Model file for the job. Use its own axes, mm. A direction names the side the tool comes from. Round coordinates to 2 decimals unless told otherwise and drop trailing zeros. Loops run counter-clockwise (first coordinate to the right, second up) from the corner with the lowest first, then second, coordinate; pieces in that order, holes last. Notation, with made-up numbers: M 88.5,49.5 L 142.5,49.5 A16 cw 142.5,69.5 Z; hole C 15,17.25 d2. An arc over 180 degrees is marked long. Use a Markdown table: item, result. Add a question column.
Q1. Tool access for faces 1 (the face through (0.3, 43.5, 32.414)), 2 (the face through (45, 0, 50)): list every direction of +Z, -Z, +X, -X, +Y, -Y with a clear straight run to the whole face (end or side of a thin tool).
Q2. Cut at B-B (y = -0.5). Give the cut face in (x, z), plus the area to 3 significant figures.
Q3. Pin check, flat tips, straight feed: pin 1 (8 mm diameter, centred on x = 15, y = 15, fed in from +Z); pin 2 (8 mm diameter, centred on x = 37.5, z = 42, fed in from -Y); pin 3 (13.5 mm diameter, centred on y = 40.5, z = 21, fed in from +X). Stop position of each tip, or through.
Q4. Cut at C-C (y = 62). Give the cut face in (x, z), plus the area to 3 significant figures.
Q5. Cut at D-D (z = 4.5). Give the cut face in (x, y), plus the area to 3 significant figures.
Q6. Cut at A-A (x = 0). Give the cut face in (y, z).
Q7. Mould opens along Y. For faces 3 (the face through (16.7, 75.7, 24)), 4 (the face through (-2.71, 44.434, 23.959)), 5 (the face through (-21.187, 46, 24)) say: +Y half, -Y half, draft (parallel to the pull), parting line (faces both ways), or undercut.
Q8. Probe line 1 (Y direction, x = 0, z = 27); line 2 (Y direction, x = 0, z = 19); line 3 (Y direction, x = -2, z = 35.5) (3 decimals). List the from-to ranges inside material, lowest first. Write a range as from..to.
from build123d import *

# Parameters (mm, degrees)
F0_W         = 100
F0_H         = 60
F1_DEPTH     = 60
F2_W         = 42.3733331263
F2_H         = 17.1486828476
F3_DEPTH     = 50
F4_R         = 12.5
F5_DEPTH     = 32.4145003611
F6_T1_DEPTH  = 185
F6_T3_DEPTH  = 225
F6_T8_DEPTH  = 225
F6_T14_DEPTH = 225
F6_T20_DEPTH = 225
F6_T27_DEPTH = 225
F6_T33_DEPTH = 225
F7_R         = 15


# Not quite as in the source:
# - a fillet or chamfer that OpenCascade refuses, or shapes differently, is made with other operations: its cross-section is extruded or revolved along the edge and cut away or added


with BuildPart() as f1:
    # F0 (on Top) → F1 (new body)
    with BuildSketch(Plane.XY):
        Rectangle(F0_W, F0_H)
    extrude(amount=F1_DEPTH)

    # F2 (on face) → F3 (join)
    with BuildSketch(Plane(origin=(0, 30, 0), x_dir=(-1, 0, 0), z_dir=(0, 1, 0))):
        with Locations((0, 23.8391589373)):
            Rectangle(F2_W, F2_H)
    extrude(amount=F3_DEPTH)

    # F4 (on face) → F5 (cut, through all)
    with BuildSketch(Plane.XY.offset(32.4135003611)):
        with Locations((0, 56.6370971501)):
            Circle(F4_R)
    extrude(amount=-F5_DEPTH, mode=Mode.SUBTRACT)

    # F6: fillet of radius 25 on 8 edges, made by hand

    # F6_s2 → F6_t1 (cut)
    with BuildSketch(Plane.XZ.offset(-92.5)):
        with BuildLine():
            ThreePointArc((-50, 35), (-42.6776695297, 52.6776695297), (-25, 60))
            Line((-25, 60), (-50, 60))
            Line((-50, 60), (-50, 35))
        make_face()
        with BuildLine():
            ThreePointArc((25, 60), (42.6776695297, 52.6776695297), (50, 35))
            Line((50, 35), (50, 60))
            Line((50, 60), (25, 60))
        make_face()
        with BuildLine():
            ThreePointArc((-50, 25), (-42.6776695297, 7.3223304703), (-25, 0))
            Line((-25, 0), (-50, 0))
            Line((-50, 0), (-50, 25))
        make_face()
        with BuildLine():
            ThreePointArc((25, 0), (42.6776695297, 7.3223304703), (50, 25))
            Line((50, 25), (50, 0))
            Line((50, 0), (25, 0))
        make_face()
    extrude(amount=F6_T1_DEPTH, mode=Mode.SUBTRACT)

    # F6_s4 → F6_t3 (cut)
    with BuildSketch(Plane.YZ.offset(-112.5)):
        with BuildLine():
            ThreePointArc((-30, 35), (-22.6776695297, 52.6776695297), (-5, 60))
            Line((-5, 60), (-30, 60))
            Line((-30, 60), (-30, 35))
        make_face()
        with BuildLine():
            ThreePointArc((30, 35), (22.6776695297, 52.6776695297), (5, 60))
            Line((5, 60), (30, 60))
            Line((30, 60), (30, 35))
        make_face()
        with BuildLine():
            ThreePointArc((-30, 25), (-22.6776695297, 7.3223304703), (-5, 0))
            Line((-5, 0), (-30, 0))
            Line((-30, 0), (-30, 25))
        make_face()
    extrude(amount=F6_T3_DEPTH, mode=Mode.SUBTRACT)


with BuildPart() as f6_tool6:
    # F6_s7 → F6_t8 (new body)
    with BuildSketch(Plane.YZ.offset(112.5)):
        with BuildLine():
            ThreePointArc((30, 25), (22.6776695297, 7.3223304703), (5, 0))
            Line((5, 0), (30, 0))
            Line((30, 0), (30, 25))
        make_face()
    extrude(amount=-F6_T8_DEPTH)

    split(bisect_by=Plane.XY.offset(15.2648175135), keep=Keep.TOP)

    split(bisect_by=Plane.YZ.offset(21.1866665632), keep=Keep.TOP)


with BuildPart() as f1_1:
    add(f1.part)

    # F6_t5: cut F6_tool6
    add(f6_tool6.part, mode=Mode.SUBTRACT)


with BuildPart() as f6_tool12:
    # F6_s13 → F6_t14 (new body)
    with BuildSketch(Plane.YZ.offset(112.5)):
        with BuildLine():
            ThreePointArc((30, 25), (22.6776695297, 7.3223304703), (5, 0))
            Line((5, 0), (30, 0))
            Line((30, 0), (30, 25))
        make_face()
    extrude(amount=-F6_T14_DEPTH)

    split(bisect_by=Plane.XY.offset(15.2648175135), keep=Keep.BOTTOM)

    split(bisect_by=Plane.YZ.offset(21.1866665632), keep=Keep.TOP)


with BuildPart() as f1_2:
    add(f1_1.part)

    # F6_t11: cut F6_tool12
    add(f6_tool12.part, mode=Mode.SUBTRACT)


with BuildPart() as f6_tool18:
    # F6_s19 → F6_t20 (new body)
    with BuildSketch(Plane.YZ.offset(112.5)):
        with BuildLine():
            ThreePointArc((30, 25), (22.6776695297, 7.3223304703), (5, 0))
            Line((5, 0), (30, 0))
            Line((30, 0), (30, 25))
        make_face()
    extrude(amount=-F6_T20_DEPTH)

    split(bisect_by=Plane.XY.offset(15.2648175135), keep=Keep.BOTTOM)

    split(bisect_by=Plane.YZ.offset(21.1866665632), keep=Keep.BOTTOM)

    split(bisect_by=Plane.YZ.offset(-21.1866665632), keep=Keep.TOP)


with BuildPart() as f1_3:
    add(f1_2.part)

    # F6_t17: cut F6_tool18
    add(f6_tool18.part, mode=Mode.SUBTRACT)


with BuildPart() as f6_tool25:
    # F6_s26 → F6_t27 (new body)
    with BuildSketch(Plane.YZ.offset(112.5)):
        with BuildLine():
            ThreePointArc((30, 25), (22.6776695297, 7.3223304703), (5, 0))
            Line((5, 0), (30, 0))
            Line((30, 0), (30, 25))
        make_face()
    extrude(amount=-F6_T27_DEPTH)

    split(bisect_by=Plane.XY.offset(15.2648175135), keep=Keep.TOP)

    split(bisect_by=Plane.YZ.offset(-21.1866665632), keep=Keep.BOTTOM)


with BuildPart() as f1_4:
    add(f1_3.part)

    # F6_t24: cut F6_tool25
    add(f6_tool25.part, mode=Mode.SUBTRACT)


with BuildPart() as f6_tool31:
    # F6_s32 → F6_t33 (new body)
    with BuildSketch(Plane.YZ.offset(112.5)):
        with BuildLine():
            ThreePointArc((30, 25), (22.6776695297, 7.3223304703), (5, 0))
            Line((5, 0), (30, 0))
            Line((30, 0), (30, 25))
        make_face()
    extrude(amount=-F6_T33_DEPTH)

    split(bisect_by=Plane.XY.offset(15.2648175135), keep=Keep.BOTTOM)

    split(bisect_by=Plane.YZ.offset(-21.1866665632), keep=Keep.BOTTOM)


with BuildPart() as f1_5:
    add(f1_4.part)

    # F6_t30: cut F6_tool31
    add(f6_tool31.part, mode=Mode.SUBTRACT)

    # F7
    f7_edges = [f1_5.edges().sort_by_distance(p)[0] for p in [
        (-21.186667, 80, 23.839159),
        (21.186667, 80, 23.839159),
    ]]
    fillet(f7_edges, radius=F7_R)


solid = f1_5.part
Checked values:
| question | item | result |
|---|---|---|
| 1 | face 1 | +Z, +X, -X, +Y |
| 1 | face 2 | +Z, +X, +Y, -Y |
| 2 | outline | M -50,25 A25 ccw -25,0 L 25,0 A25 ccw 50,25 L 50,35 A25 ccw 25,60 L -25,60 A25 ccw -50,35 Z |
| 2 | area | 5,460 mm^2 |
| 3 | pin 1 | stops at z = 59.27 |
| 3 | pin 2 | stops at y = -29.82 |
| 3 | pin 3 | stops at x = 21.19 |
| 4 | outline | M -21.19,15.26 L -11.29,15.26 L -11.29,32.41 L -21.19,32.41 Z; M 11.29,15.26 L 21.19,15.26 L 21.19,32.41 L 11.29,32.41 Z |
| 4 | area | 339 mm^2 |
| 5 | outline | M -39.31,-19.31 L 39.31,-19.31 L 39.31,19.31 L -39.31,19.31 Z |
| 5 | area | 3,040 mm^2 |
| 6 | outline | M -30,25 A25 ccw -5,0 L 5,0 A25 ccw 28.03,15.26 L 44.14,15.26 L 44.14,32.41 L 30,32.41 L 30,35 A25 ccw 5,60 L -5,60 A25 ccw -30,35 Z; M 69.14,15.26 L 80,15.26 L 80,32.41 L 69.14,32.41 Z |
| 7 | face 3 | +Y half |
| 7 | face 4 | undercut |
| 7 | face 5 | draft |
| 8 | line 1 | y = -30..44.14, 69.14..80 |
| 8 | line 2 | y = -29.27..44.14, 69.14..80 |
| 8 | line 3 | y = -29.995..29.995 |
